Geometry: final body of the model. Coordinates: model frame, mm. Face numbers are marked on the shaded views. A direction names the side the tool comes from. Give positions to 0.01 mm unless a question says otherwise; leave off trailing zeros. Order: outer loops, then holes, each group sorted by start corner. A loop starts at its lowest first (then second) coordinate and runs counter-clockwise, first axis right, second up. Notation, with made-up numbers: (28, 57.25) -> (49, 57.25) arc R13 ccw to (49, 80.25) -> close; hole circle Ø5 at (36, 72). An arc over 180 degrees is marked (long way). Answer in a Markdown table with one row per item. Add a question column.
Q1. Set-up query: the marked faces 1 and 2. Return all of +Z, -Z, +X, -X, +Y, -Y with unobstructed straight access to the full face (end or side cutting, diameter ignored); none if empty.
Q2. Cut plane A-A on x = 15. Return the cut outline in (y, z), and give its area (3 significant figures).
Q3. Cut plane D-D on z = 0. Return the cut outline in (x, y), and give its area (3 significant figures).
Q4. Cut plane B-B on z = -18. Return the cut outline in (x, y).
Q5. Cut plane C-C on x = 0. Return the cut outline in (y, z).
Q6. Contact query for flat-ended pins moving along their axis: P1, Ø3.5, axis at x = 0, z = -18, coming from the +Y side; P2, Ø5, axis at x = -10, y = 10, coming from the -Z side; P3, Ø3, axis at x = -16.5, z = 2, coming from the -Y side; P4, Ø0.5, axis at x = 15.5, y = 14.5, coming from the +Z side. Output: stop coordinate, or through.
Q7. Line query: line 1 along X through (y, z) = (15.7, 0); line 2 along Y through (x, z) = (-15, 34); line 3 along X through (y, z) = (20, -18). Output: solid intervals per line, ascending. Write a range as from..to.
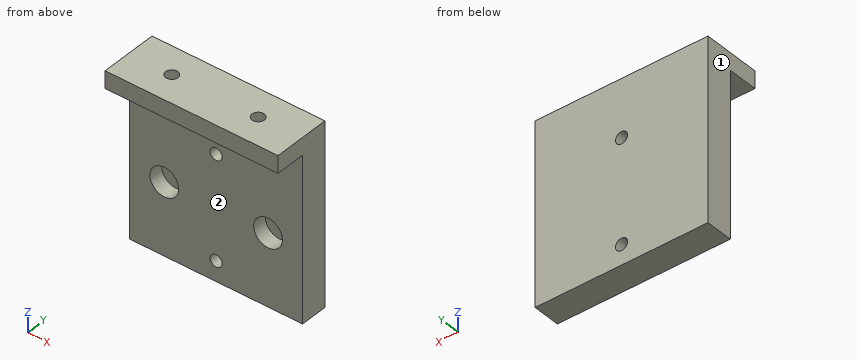
from build123d import *

# Parameters (mm, degrees)
SK_TOP_W              = 60
SK_TOP_H              = 63
EX_TOP_DEPTH          = 9.5
SK_BACKWALL_W         = 60
SK_BACKWALL_H         = 6
EX_BACKWALL_DEPTH     = 10.5
SK_RAILBOLTS_R        = 2.15
CUT_RAILBOLTS_DEPTH   = 8
SK_GUIDEPINS_R        = 2.1
CUT_GUIDEPINS_DEPTH   = 9.5
SK_SPRINGSEATS_R      = 5
CUT_SPRINGSEATS_DEPTH = 5


with BuildPart() as part:
    # SK_Top → EX_Top (new body)
    with BuildSketch(Plane(origin=(0, 14, 0), x_dir=(1, 0, 0), z_dir=(0, 1, 0))):
        with Locations((0, -6.5)):
            Rectangle(SK_TOP_W, SK_TOP_H)
    extrude(amount=EX_TOP_DEPTH)

    # SK_BackWall → EX_BackWall (add)
    with BuildSketch(Plane(origin=(0, 3.5, 0), x_dir=(1, 0, 0), z_dir=(0, 1, 0))):
        with Locations((0, -35)):
            Rectangle(SK_BACKWALL_W, SK_BACKWALL_H)
    extrude(amount=EX_BACKWALL_DEPTH)

    # SK_RailBolts → CUT_RailBolts (cut)
    with BuildSketch(Plane.XY.offset(38)):
        with Locations((15, 13.5)):
            Circle(SK_RAILBOLTS_R)
        with Locations((-15, 13.5)):
            Circle(SK_RAILBOLTS_R)
    extrude(amount=-CUT_RAILBOLTS_DEPTH, mode=Mode.SUBTRACT)

    # SK_GuidePins → CUT_GuidePins (cut)
    with BuildSketch(Plane(origin=(0, 14, 0), x_dir=(1, 0, 0), z_dir=(0, 1, 0))):
        with Locations(Location((0, -18, 0), (0, 0, 270))):
            Circle(SK_GUIDEPINS_R)
        with Locations(Location((0, 18, 0), (0, 0, 270))):
            Circle(SK_GUIDEPINS_R)
    extrude(amount=CUT_GUIDEPINS_DEPTH, mode=Mode.SUBTRACT)

    # SK_SpringSeats → CUT_SpringSeats (cut)
    with BuildSketch(Plane(origin=(0, 14, 0), x_dir=(1, 0, 0), z_dir=(0, 1, 0))):
        with Locations(Location((18, 0, 0), (0, 0, 270))):
            Circle(SK_SPRINGSEATS_R)
        with Locations(Location((-18, 0, 0), (0, 0, 270))):
            Circle(SK_SPRINGSEATS_R)
    extrude(amount=CUT_SPRINGSEATS_DEPTH, mode=Mode.SUBTRACT)


solid = part.part
Completed:
| question | item | result |
|---|---|---|
| 1 | face 1 | +Z, -Z, -X, +Y, -Y |
| 1 | face 2 | -Z, +X, -X, -Y |
| 2 | outline | (3.5, 32) -> (11.35, 32) -> (11.35, 38) -> (3.5, 38) -> close; (14, -25) -> (23.5, -25) -> (23.5, 38) -> (15.65, 38) -> (15.65, 30) -> (14, 30) -> (14, 4) -> (19, 4) -> (19, -4) -> (14, -4) -> close |
| 2 | area | 592 mm² |
| 3 | outline | (-30, 14) -> (-23, 14) -> (-23, 19) -> (-13, 19) -> (-13, 14) -> (13, 14) -> (13, 19) -> (23, 19) -> (23, 14) -> (30, 14) -> (30, 23.5) -> (-30, 23.5) -> close |
| 3 | area | 470 mm² |
| 4 | outline | (-30, 14) -> (-2.1, 14) -> (-2.1, 23.5) -> (-30, 23.5) -> close; (2.1, 14) -> (30, 14) -> (30, 23.5) -> (2.1, 23.5) -> close |
| 5 | outline | (3.5, 32) -> (14, 32) -> (14, 20.1) -> (23.5, 20.1) -> (23.5, 38) -> (3.5, 38) -> close; (14, -25) -> (23.5, -25) -> (23.5, -20.1) -> (14, -20.1) -> close; (14, -15.9) -> (23.5, -15.9) -> (23.5, 15.9) -> (14, 15.9) -> close |
| 6 | P1 | passes through |
| 6 | P2 | stops at z = 32 |
| 6 | P3 | stops at y = 19 |
| 6 | P4 | stops at z = 30 |
| 7 | line 1 | x = -30..-23, -13..13, 23..30 |
| 7 | line 2 | y = 3.5..11.35, 15.65..23.5 |
| 7 | line 3 | x = -30..-2.1, 2.1..30 |
